```python
from build123d import *

# Parameters (mm, degrees)
SKETCH1_W           = 105
SKETCH1_H           = 4
SKETCH1_W_2         = 2
SKETCH1_H_2         = 9.8
BOSS_EXTRUDE1_DEPTH = 12.5
SKETCH2_W           = 8
SKETCH2_H           = 10
SKETCH2_R           = 1.55
BOSS_EXTRUDE2_DEPTH = 2
SKETCH4_W           = 8
SKETCH4_H           = 10
SKETCH4_R           = 1.55
BOSS_EXTRUDE3_DEPTH = 2
SKETCH5_W           = 101
SKETCH5_H           = 2
CUT_EXTRUDE1_DEPTH  = 1.8
SKETCH6_W           = 101
SKETCH6_H           = 2
CUT_EXTRUDE2_DEPTH  = 1.8


with BuildPart() as part:
    # Sketch1 → Boss-Extrude1 (new body, symmetric)
    with BuildSketch(Plane(origin=(0, 0, 0), x_dir=(0, 0, -1), z_dir=(1, 0, 0))):
        Rectangle(SKETCH1_W, SKETCH1_H)
        Polygon((-52.5, 63.2), (-52.5, 2), (-48.5, 2), (-48.5, 63.2), (-50.5, 63.2), align=None)
        Polygon((48.5, 63.2), (48.5, 2), (52.5, 2), (52.5, 63.2), (50.5, 63.2), align=None)
        with Locations((-49.5, 68.1)):
            Rectangle(SKETCH1_W_2, SKETCH1_H_2)
        with Locations((49.5, 68.1)):
            Rectangle(SKETCH1_W_2, SKETCH1_H_2)
    extrude(amount=BOSS_EXTRUDE1_DEPTH, both=True)

    # Sketch2 → Boss-Extrude2 (add)
    with BuildSketch(Plane.XY.offset(-48.5)):
        with Locations((-16.5, 16)):
            Rectangle(SKETCH2_W, SKETCH2_H)
        with Locations((-16.5, 16)):
            Circle(SKETCH2_R, mode=Mode.SUBTRACT)
        with Locations((-16.5, 44)):
            Rectangle(SKETCH2_W, SKETCH2_H)
        with Locations((-16.5, 44)):
            Circle(SKETCH2_R, mode=Mode.SUBTRACT)
        with Locations((16.5, 16)):
            Rectangle(SKETCH2_W, SKETCH2_H)
        with Locations((16.5, 16)):
            Circle(SKETCH2_R, mode=Mode.SUBTRACT)
        with Locations((16.5, 44)):
            Rectangle(SKETCH2_W, SKETCH2_H)
        with Locations((16.5, 44)):
            Circle(SKETCH2_R, mode=Mode.SUBTRACT)
    extrude(amount=-BOSS_EXTRUDE2_DEPTH)

    # Sketch4 → Boss-Extrude3 (add)
    with BuildSketch(Plane(origin=(0, 0, 48.5), x_dir=(-1, 0, 0), z_dir=(0, 0, -1))):
        with Locations((-16.5, 16)):
            Rectangle(SKETCH4_W, SKETCH4_H)
        with Locations((-16.5, 16)):
            Circle(SKETCH4_R, mode=Mode.SUBTRACT)
        with Locations((-16.5, 44)):
            Rectangle(SKETCH4_W, SKETCH4_H)
        with Locations((-16.5, 44)):
            Circle(SKETCH4_R, mode=Mode.SUBTRACT)
        with Locations((16.5, 16)):
            Rectangle(SKETCH4_W, SKETCH4_H)
        with Locations((16.5, 16)):
            Circle(SKETCH4_R, mode=Mode.SUBTRACT)
        with Locations((16.5, 44)):
            Rectangle(SKETCH4_W, SKETCH4_H)
        with Locations((16.5, 44)):
            Circle(SKETCH4_R, mode=Mode.SUBTRACT)
    extrude(amount=-BOSS_EXTRUDE3_DEPTH)

    # Sketch5 → Cut-Extrude1 (cut)
    with BuildSketch(Plane.ZY.offset(12.5)):
        Polygon((-50.5, 63.2), (-52.5, 63.2), (-52.5, -2), (-50.5, -2), (-50.5, 0), (-50.5, 11), (-50.5, 21), (-50.5, 39), (-50.5, 49), align=None)
        with Locations((0, -1)):
            Rectangle(SKETCH5_W, SKETCH5_H)
        Polygon((50.5, 0), (50.5, -2), (52.5, -2), (52.5, 63.2), (50.5, 63.2), (50.5, 49), (50.5, 39), (50.5, 21), (50.5, 11), align=None)
    extrude(amount=-CUT_EXTRUDE1_DEPTH, mode=Mode.SUBTRACT)

    # Sketch6 → Cut-Extrude2 (cut)
    with BuildSketch(Plane(origin=(12.5, 0, 0), x_dir=(0, 0, -1), z_dir=(1, 0, 0))):
        Polygon((-50.5, 0), (-50.5, 63.2), (-52.5, 63.2), (-52.5, -2), (-50.5, -2), align=None)
        with Locations((0, -1)):
            Rectangle(SKETCH6_W, SKETCH6_H)
        Polygon((50.5, 63.2), (50.5, 0), (50.5, -2), (52.5, -2), (52.5, 63.2), align=None)
    extrude(amount=-CUT_EXTRUDE2_DEPTH, mode=Mode.SUBTRACT)


solid = part.part
```
Design review of the part built by this model. Coordinates are the model's own, in mm. A direction names the side the tool comes from. Round coordinates to 2 decimals unless told otherwise and drop trailing zeros. Order: outer loops, then holes, each group sorted by start corner. A loop starts at its lowest first (then second) coordinate and runs counter-clockwise, first axis right, second up. Notation, with made-up numbers: M 69,19 L 123,19 A17 cw 123,38 Z; hole C -29,88.25 d3. An arc over 180 degrees is marked long. Put each result on its own line as item: value.
Q1. Consider section C-C (y = 7.5). State the section outline as (x, z) points.
Reported:
outline: M -12.5,-50.5 L -10.7,-50.5 L -10.7,-52.5 L 10.7,-52.5 L 10.7,-50.5 L 12.5,-50.5 L 12.5,-48.5 L -12.5,-48.5 Z; M -12.5,48.5 L 12.5,48.5 L 12.5,50.5 L 10.7,50.5 L 10.7,52.5 L -10.7,52.5 L -10.7,50.5 L -12.5,50.5 Z
Q2. To check wall thickness, follow line 1 (Y direction, x = 16.5, z = -49.85); line 2 (Z direction, x = 12, y = 32.5); line 3 (Z direction, x = 8, y = 30.5). State the ranges of each line that lie inside material, in increasing order.
Reported:
line 1: 11 to 14.45, 17.55 to 21, 39 to 42.45, 45.55 to 49
line 2: -50.5 to -48.5, 48.5 to 50.5
line 3: -52.5 to -48.5, 48.5 to 52.5
Q3. Machinability: for faces 4 (the face through (-12.5, 1, 8)), 5 (the face through (0, 37, 48.5)), 6 (the face through (16.836, 42.487, 49.486)), which of the approach directions +Z, -Z, +X, -X, +Y, -Y give a long, thin tool a straight path to every point of the face, cutting with its end or side? Answer none if there is none.
Reported:
face 4: +Z, -Z, -X, -Y
face 5: +X, -X, +Y
face 6: +Z, -Z
Q4. Consider section D-D (z = 35). State the section outline as (x, y) points, and give its area (3 significant figures).
Reported:
outline: M -12.5,0 L -10.7,0 L -10.7,-2 L 10.7,-2 L 10.7,0 L 12.5,0 L 12.5,2 L -12.5,2 Z
area: 92.8 mm²
Q5. Draft analysis for pull direction Y (two halves, no side actions). For faces 1 (the face through (12.5, 1, 8)), 2 (the face through (16.164, 42.487, -49.486)), 3 (the face through (0, 2, 1)), state which applies: released by +Y, released by -Y, zero draft, split by the parting line, or undercut.
Reported:
face 1: zero draft
face 2: undercut
face 3: released by +Y
Q6. Insertion check: pin 1 Ø2 at (x, z) = (-17, 50) entering from +Y; pin 2 Ø0.6 at (x, z) = (17, -49) entering from -Y; pin 3 Ø0.5 at (x, z) = (11.5, 22.5) entering from -Y; pin 4 Ø1.4 at (x, z) = (-11, -9) entering from -Y. Each pin has a flat end and moves straight along its axis. Give the tip position at first contact, or say it passes through.
Reported:
pin 1: y = 49
pin 2: y = 11
pin 3: y = 0
pin 4: y = -2
Q7. Consider section A-A (y = 44). State how many separate pieces and enclosed holes the cut face has, and give its area (3 significant figures).
Reported:
separate pieces: 6
enclosed holes: 0
area: 225 mm²
